from build123d import *

# Parameters (mm, degrees)
RESSALTO_EXTRUS_O1_DEPTH = 175
FILETE1_R                = 0.5
ESBO_O2_R                = 1.5
CORTE_EXTRUS_O1_DEPTH    = 190.446275038


with BuildPart() as part:
    # Esboço1 → Ressalto-extrusão1 (new body)
    with BuildSketch(Plane(origin=(0, 0, 0), x_dir=(-1, 0, 0), z_dir=(0, 0, -1))):
        Polygon((67.502122675, -1.443375673), (70.002122675, -2.886751346), (72.502122675, -1.443375673), (72.502122675, 1.443375673), (70.002122675, 2.886751346), (67.502122675, 1.443375673), align=None)
    extrude(amount=-RESSALTO_EXTRUS_O1_DEPTH)

    # Filete1
    filete1_edges = [part.edges().sort_by_distance(p)[0] for p in [
        (-71.252122675, -2.165063509, 175),
        (-72.502122675, 0, 175),
        (-71.252122675, 2.165063509, 175),
        (-68.752122675, 2.165063509, 175),
        (-67.502122675, 0, 175),
        (-68.752122675, 2.165063509, 0),
        (-71.252122675, 2.165063509, 0),
        (-72.502122675, 0, 0),
        (-71.252122675, -2.165063509, 0),
        (-68.752122675, -2.165063509, 0),
        (-67.502122675, 0, 0),
        (-68.752122675, -2.165063509, 175),
    ]]
    fillet(filete1_edges, radius=FILETE1_R)

    # Esboço2 → Corte-extrusão1 (cut, through all)
    with BuildSketch(Plane.XY.offset(175)):
        with Locations((-70.002122675, 0)):
            Circle(ESBO_O2_R)
    extrude(amount=-CORTE_EXTRUS_O1_DEPTH, mode=Mode.SUBTRACT)


solid = part.part
The listing builds one solid part. Answer for the finished solid, in the listing's coordinates (mm). Round coordinates to 2 decimals unless told otherwise and drop trailing zeros. Write each loop counter-clockwise with the first axis right and the second up, starting at its lowest first coordinate (ties: lowest second). Pieces come first, ordered by that corner, then holes. Notation, with made-up numbers: M 80.5,50 L 88.5,50 A20 cw 88.5,73 Z; hole C -10.75,-10 d9. An arc over 180 degrees is marked long. Write each question's results on one line, items separated by ' | '. Start each with the question number.
(1) This flat-tipped pin is pushed along its axis until it touches: P1, Ø3, axis at x = -71, z = 124, coming from the +Y side. Where does it stop, or does it pass through?
(2) Determine the mould class of faces 1 (the cylindrical face through (-68.57, 0.45, 88.72)), 2 (the flat face through (-67.502, 0, 86)) for opening direction Y: +Y half, -Y half, draft (parallel to the pull), parting line (faces both ways), or undercut.
(3) Find the intervals of material crossed by line 1 (X direction, y = -0.25, z = 39.5); line 2 (Y direction, x = -68.7, z = 26); line 3 (Y direction, x = -70.55, z = 64), in increasing order.
(4) The part is cut by section A-A, the plane y = 0. Write down the section's boundary in (x, z), and give its area (3 significant figures).
(5) The part is cut by section B-B, the plane z = 56.5. Write down the section's boundary in (x, y), and give its area (3 significant figures).
Worked answers:
1) P1: stops at y = 2.89
2) face 1: undercut | face 2: draft
3) line 1: x = -72.5 to -71.48, -68.52 to -67.5 | line 2: y = -2.13 to -0.74, 0.74 to 2.13 | line 3: y = -2.57 to -1.4, 1.4 to 2.57
4) outline: M -72.5,0.5 A0.5 ccw -72,0 L -71.5,0 L -71.5,175 L -72,175 A0.5 ccw -72.5,174.5 Z; M -68.5,0 L -68,0 A0.5 ccw -67.5,0.5 L -67.5,174.5 A0.5 ccw -68,175 L -68.5,175 Z | area: 350 mm²
5) outline: M -72.5,-1.44 L -70,-2.89 L -67.5,-1.44 L -67.5,1.44 L -70,2.89 L -72.5,1.44 Z; hole C -70,0 d3 | area: 14.6 mm²
